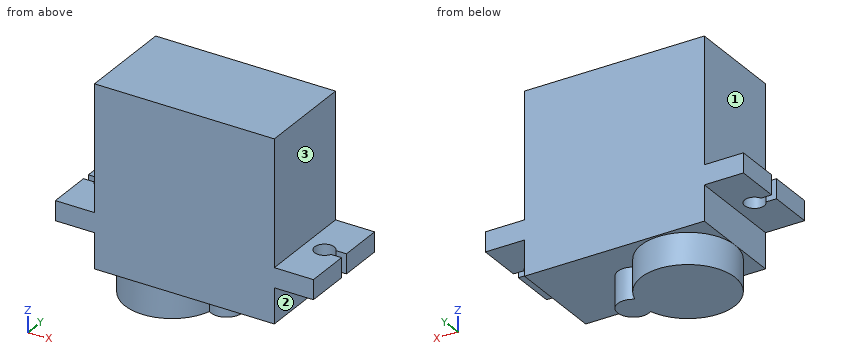
Autodesk Inventor part; units mm, degrees
ref_plane "YZ Plane" through (0, 0, 0) normal (1, 0, 0) x (0, 1, 0)
ref_plane "XZ Plane" through (0, 0, 0) normal (0, 1, 0) x (-1, 0, 0)
ref_plane "XY Plane" through (0, 0, 0) normal (0, 0, 1) x (1, 0, 0)
sketch "Sketch1" plane through (0, 0, 0) normal (0, 1, 0) x (-1, 0, 0)
  line L0 (0, 0) -> (-23, 0)
  line L1 (-23, 0) -> (-23, 23)
  line L2 (-23, 23) -> (0, 23)
  line L3 (0, 23) -> (0, 0)
  line L4 (-23, 0) -> (-23, 7)
  line L5 (-23, 7) -> (-28, 7)
  line L6 (-28, 7) -> (-28, 4.5)
  line L7 (-28, 4.5) -> (-23, 4.5)
  line L8 (0, 7) -> (5, 7)
  line L9 (5, 7) -> (5, 4.5)
  line L10 (5, 4.5) -> (0, 4.5)
  dimension "d0" = 23
  dimension "d1" = 23
  dimension "d2" = 7
  dimension "d3" = 5
  dimension "d4" = 2.5
extrude "Extrusion1" add sketch "Sketch1" along normal blind 12.5
sketch "Sketch2" plane through (23, 0, 0) normal (0, 0, -1) x (-1, 0, 0)
  line L0 (23, 0) -> (23, 6.25)
  arc A0 (11.2156, 4.6561) -> (11.2214, 7.865) centre (17, 6.25) ccw
  arc A1 (11.2214, 7.865) -> (11.2156, 4.6561) centre (10.0244, 6.2627) ccw
extrude "Extrusion2" add sketch "Sketch2" along normal blind 4
sketch "Sketch3" plane through (28, 0, 4.5) normal (0, 0, -1) x (-1, 0, 0)
  line L0 (0, 0) -> (0, 12.5)
  line L1 (0, 6.25) -> (2.5, 6.25)
  circle A0 centre (2.5, 6.25) radius 1.25
  point P0 (28, 0)
  dimension "d11" = 2.5
  dimension "d12" = 2.5
extrude "Extrusion3" cut sketch "Sketch3" against normal blind 2.5
sketch "Sketch4" plane through (28, 0, 4.5) normal (0, 0, -1) x (-1, 0, 0)
  circle A0 centre (2.5, 6.25) radius 1.25
  line L0 (0, 0) -> (0, 12.5)
  line L1 (1.25, 5.75) -> (0, 5.75)
  line L2 (1.25, 6.75) -> (0, 6.75)
  line L3 (1.25, 6.75) -> (1.3544, 6.75)
  line L4 (1.25, 5.75) -> (1.3544, 5.75)
  line L5 (0, 6.75) -> (0, 5.75)
  arc A1 (1.25, 6.25) -> (1.3544, 6.75) centre (2.5, 6.25) ccw
  point P0 (28, 0)
extrude "Extrusion4" cut sketch "Sketch4" against normal blind 2.5 contours A0 L4 L1 L0 L2 L3
sketch "Sketch5" plane through (28, 0, 4.5) normal (0, 0, -1) x (-1, 0, 0)
  line L0 (5, 0) -> (28, 0)
  line L1 (16.5, 0) -> (16.5, 12.5)
  line L2 (5, 12.5) -> (28, 12.5)
  arc A0 (1.3544, 5.75) -> (1.3544, 6.75) centre (2.5, 6.25) ccw
  line L3 (1.3544, 6.75) -> (0, 6.75)
  line L4 (1.3544, 6.75) -> (0, 6.75)
  line L5 (0, 6.75) -> (0, 5.75)
  line L6 (0, 5.75) -> (1.3544, 5.75)
  arc A1 (31.6456, 6.75) -> (31.6456, 5.75) centre (30.5, 6.25) ccw
  line L7 (31.6456, 6.75) -> (33, 6.75)
  line L8 (33, 6.75) -> (33, 5.75)
  line L9 (33, 5.75) -> (31.6456, 5.75)
extrude "Extrusion5" cut sketch "Sketch5" against normal blind 2.5 contours L7 L8 L9 A1
properties part number "Micro servo"
The model under review builds one solid part; all positions refer to its coordinate system, in mm. Face numbers are marked on the shaded views. A direction names the side the tool comes from. Round coordinates to 2 decimals unless told otherwise and drop trailing zeros. Loops run counter-clockwise (first coordinate to the right, second up) from the corner with the lowest first, then second, coordinate; pieces in that order, holes last. Notation, with made-up numbers: M -34,39.25 L -29,39.25 A23 cw -29,77.25 Z; hole C 88.25,50 d5. An arc over 180 degrees is marked long. Put each result on its own line as item: value.
Q1. Consider section A-A, the plane x = 25.5. Give the boundary of the cut face in (y, z).
Result set:
outline: M 0,4.5 L 5,4.5 L 5,7 L 0,7 Z; M 7.5,4.5 L 12.5,4.5 L 12.5,7 L 7.5,7 Z
Q2. For pin 1 (8 mm diameter, centred on x = 1, z = 11, fed in from -Y); pin 2 (6 mm diameter, centred on y = 8, z = 13, fed in from +X); pin 3 (2.5 mm diameter, centred on x = -2.5, y = 7.5, fed in from -Z); pin 4 (5 mm diameter, centred on y = 4.5, z = 1.5, fed in from -X), all flat-tipped, find the tip position at first contact; note any pin that passes through.
Result set:
pin 1: stops at y = 0
pin 2: stops at x = 23
pin 3: stops at z = 4.5
pin 4: stops at x = 0
Q3. Consider section D-D, the plane z = 9.5. Give the boundary of the cut face in (x, y).
Result set:
outline: M 0,0 L 23,0 L 23,12.5 L 0,12.5 Z
Q4. To check wall thickness, follow L1, parallel to Y at x = -2.5, z = 6.1; L2, parallel to Z at x = 26.5, y = 4; L3, parallel to X at y = 10.25, z = 10. State the ranges of each line that lie inside material, in increasing order.
Result set:
L1: y = 0 to 5, 7.5 to 12.5
L2: z = 4.5 to 7
L3: x = 0 to 23
Q5. Machinability: for the marked faces 1, 2 and 3, which of the approach directions +Z, -Z, +X, -X, +Y, -Y give a long, thin tool a straight path to every point of the face, cutting with its end or side? Answer none if there is none.
Result set:
face 1: +Z, -X, +Y, -Y
face 2: -Z, +X, +Y, -Y
face 3: +Z, +X, +Y, -Y
Q6. Consider section B-B, the plane y = 3.75. Give the boundary of the cut face in (x, z).
Result set:
outline: M -5,4.5 L 0,4.5 L 0,0 L 0.55,0 L 0.55,-4 L 11.45,-4 L 11.45,0 L 23,0 L 23,4.5 L 28,4.5 L 28,7 L 23,7 L 23,23 L 0,23 L 0,7 L -5,7 Z
Q7. Consider section C-C, the plane x = 9. Give the boundary of the cut face in (y, z), then the cut area to 3 significant figures.
Result set:
outline: M 0,0 L 1.05,0 L 1.05,-4 L 11.45,-4 L 11.45,0 L 12.5,0 L 12.5,23 L 0,23 Z
area: 329 mm²
